Work out the finished part from the listing and answer in its coordinate system (mm). Face numbers are marked on the shaded views. A direction names the side the tool comes from. Round coordinates to 2 decimals unless told otherwise and drop trailing zeros. Loops run counter-clockwise (first coordinate to the right, second up) from the corner with the lowest first, then second, coordinate; pieces in that order, holes last. Notation, with made-up numbers: (82.25, -3) -> (88.25, -3) arc R7 cw to (88.25, 4) -> close; hole circle Ø7 at (12, 39.25). An arc over 180 degrees is marked (long way). Use one line per item in the form item = value.
```python
from build123d import *

# Parameters (mm, degrees)
F1_DEPTH = 10.5
F3_DEPTH = 25
F2_W     = 3.2
F2_H     = 23
F4_DEPTH = 15
F5_SIZE  = 5
F8_DEPTH = 21


with BuildPart() as f1:
    # F0 (on Right) → F1 (new body)
    with BuildSketch(Plane.YZ):
        Polygon((0, 0), (0, -23), (-46.5, -23), (-51, -23), (-58, -23), (-58, -30), (7, -30), (7, 0), align=None)
    extrude(amount=F1_DEPTH)

    # F2 (on face) → F3 (cut)
    with BuildSketch(Plane(origin=(0, 7, 0), x_dir=(-1, 0, 0), z_dir=(0, 1, 0))):
        with BuildLine():
            Line((-4.9, -13.8), (-4.9, -3.8))
            ThreePointArc((-4.9, -3.8), (-6.7, -2), (-8.5, -3.8))
            Line((-8.5, -3.8), (-8.5, -13.8))
            ThreePointArc((-8.5, -13.8), (-6.7, -15.6), (-4.9, -13.8))
        make_face()
    extrude(amount=-F3_DEPTH, mode=Mode.SUBTRACT)

    # F2 (on face) → F4 (join)
    with BuildSketch(Plane(origin=(0, 7, 0), x_dir=(-1, 0, 0), z_dir=(0, 1, 0))):
        with Locations((-1.6, -11.5)):
            Rectangle(F2_W, F2_H)
    extrude(amount=-F4_DEPTH)

    # F5
    f5_edges = [f1.edges().sort_by_distance(p)[0] for p in [
        (1.6, -8, -23),
        (1.6, -8, 0),
        (6.85, 0, -23),
    ]]
    chamfer(f5_edges, length=F5_SIZE)

    # F6: F1 across face


with BuildPart() as f1_1:
    add(f1.part)
    add(f1.part.mirror(Plane(origin=(0, -14.7708333333, -20.3385416667), x_dir=(0, -1, 0), z_dir=(-1, 0, 0))))

    # F7 (on face) → F8 (join, symmetric)
    with BuildSketch(Plane(origin=(-10.5, 0, 0), x_dir=(0, -1, 0), z_dir=(-1, 0, 0))):
        Polygon((34, -30), (58, -30), (58, -21), (56, -21), (56, -23), (36, -23), (36, -21), (34, -21), align=None)
    extrude(amount=F8_DEPTH, both=True)


solid = f1_1.part
```
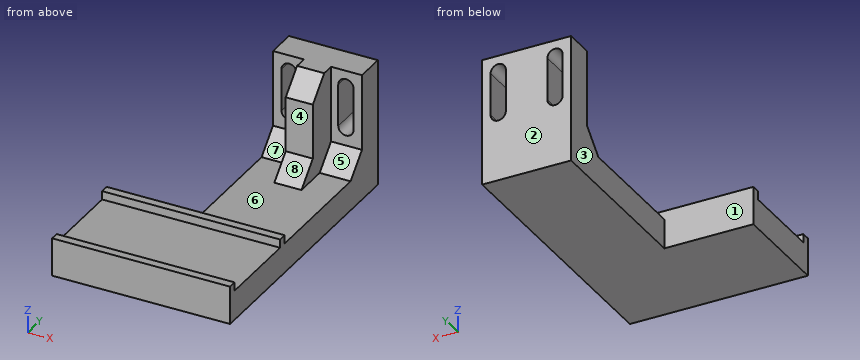
(1) For a pull along Y with two mould halves and no side action, classify the marked faces 1, 2, 3 and 4 as +Y half, -Y half, draft (parallel to the pull), parting line (faces both ways), or undercut.
Completed:
face_1 = undercut
face_2 = +Y half
face_3 = draft
face_4 = -Y half
(2) For the marked faces 5, 6, 7 and 8, determine the directions among +Z, -Z, +X, -X, +Y, -Y from which every point of the face is accessible in a straight line to the end or side of a thin tool.
Completed:
face_5 = +Z, +X
face_6 = +Z
face_7 = +Z, -X
face_8 = +Z, +X, -X
(3) Find section A-A, the plane z = -6.25. Write down the section's boundary in (x, y).
Completed:
outline = (-10.5, 0) -> (-8.5, 0) -> (-8.5, 7) -> (-10.5, 7) -> close; (-4.9, 0) -> (-3.2, 0) -> (-3.2, -8) -> (3.2, -8) -> (3.2, 0) -> (4.9, 0) -> (4.9, 7) -> (-4.9, 7) -> close; (8.5, 0) -> (10.5, 0) -> (10.5, 7) -> (8.5, 7) -> close
(4) Find section D-D, the plane x = 0. Write down the section's boundary in (y, z), then the cut area to 3 significant figures.
Completed:
outline = (-58, -30) -> (7, -30) -> (7, 0) -> (-3, 0) -> (-8, -5) -> (-8, -18) -> (-13, -23) -> (-34, -23) -> (-34, -21) -> (-36, -21) -> (-36, -23) -> (-56, -23) -> (-56, -21) -> (-58, -21) -> close
area = 808 mm2
(5) Find section C-C, the plane y = -6.5. Write down the section's boundary in (x, z), then the cut area to 3 significant figures.
Completed:
outline = (-10.5, -30) -> (10.5, -30) -> (10.5, -23) -> (3.2, -23) -> (3.2, -3.5) -> (-3.2, -3.5) -> (-3.2, -23) -> (-10.5, -23) -> close
area = 272 mm2
(6) Consider L1, parallel to X at y = 2, z = -10.5; L2, parallel to Z at x = -2.5, y = -49.5; L3, parallel to Y at x = -2.5, z = -6.5. Determine where each line is inside the solid, lowest interval first.
Completed:
L1 = -10.5 to -8.5, -4.9 to 4.9, 8.5 to 10.5
L2 = -30 to -23
L3 = -8 to 7
(7) Given P1, Ø3, axis at x = -3, y = -46, coming from the +Z side; P2, Ø2, axis at x = -14, z = -21.5, coming from the +Y side; P3, Ø6, axis at x = -8, z = -11.5, coming from the -Y side; P4, Ø12, axis at x = -17.5, y = -22.5, coming from the -Z side, each flat-ended and moving along its own axis, determine where each tip first touches the part or whether it passes through.
Completed:
P1 = -23
P2 = -34
P3 = 0
P4 = through
(8) Find section B-B, the plane x = -6.7. Write down the section's boundary in (y, z).
Completed:
outline = (-58, -30) -> (7, -30) -> (7, -15.6) -> (0, -15.6) -> (0, -18) -> (-5, -23) -> (-34, -23) -> (-34, -21) -> (-36, -21) -> (-36, -23) -> (-56, -23) -> (-56, -21) -> (-58, -21) -> close; (0, -2) -> (7, -2) -> (7, 0) -> (0, 0) -> close
